Model file for the job. Use its own axes, mm. A direction names the side the tool comes from. Give positions to 0.01 mm unless a question says otherwise; leave off trailing zeros. Order: outer loops, then holes, each group sorted by start corner. A loop starts at its lowest first (then second) coordinate and runs counter-clockwise, first axis right, second up. Notation, with made-up numbers: (-31.75, 9.25) - (8.25, 9.25) arc R21 cw to (8.25, 45.25) - close; hole circle Ø9 at (32.25, 82.25). An arc over 180 degrees is marked (long way). Return JSON: item names as keys, results as strings. Group by question number.
from build123d import *

# Parameters (mm, degrees)
BOSS_EXTRUDE1_DEPTH      = 30
BOSS_EXTRUDE2_DEPTH      = 6.5
BOSS_EXTRUDE2_DEPTH_BACK = 6.5


with BuildPart() as part:
    # Sketch1 → Boss-Extrude1 (new body)
    with BuildSketch(Plane(origin=(0, 0, 0), x_dir=(1, 0, 0), z_dir=(0, 1, 0))):
        with BuildLine():
            Line((0, 66.57), (260, 66.57))
            ThreePointArc((260, 66.57), (326.57, 0), (260, -66.57))
            Line((260, -66.57), (0, -66.57))
            ThreePointArc((0, -66.57), (-66.57, 0), (0, 66.57))
        make_face()
        with BuildLine():
            Line((0, 58.57), (260, 58.57))
            ThreePointArc((260, 58.57), (318.57, 0), (260, -58.57))
            Line((260, -58.57), (0, -58.57))
            ThreePointArc((0, -58.57), (-58.57, 0), (0, 58.57))
        make_face(mode=Mode.SUBTRACT)
    extrude(amount=BOSS_EXTRUDE1_DEPTH)

    # Sketch2 → Boss-Extrude2 (add, two sides: drawn at the far end of the back side and taken through both)
    with BuildSketch(Plane(origin=(0, 15, 0), x_dir=(-1, 0, 0), z_dir=(0, -1, 0)).offset(-BOSS_EXTRUDE2_DEPTH_BACK)):
        with BuildLine():
            Line((0, -58.57), (-260, -58.57))
            ThreePointArc((-260, -58.57), (-318.57, 0), (-260, 58.57))
            Line((-260, 58.57), (0, 58.57))
            ThreePointArc((0, 58.57), (58.57, 0), (0, -58.57))
        make_face()
        with BuildLine():
            Line((0, -50.57), (-260, -50.57))
            ThreePointArc((-260, -50.57), (-310.57, 0), (-260, 50.57))
            Line((-260, 50.57), (0, 50.57))
            ThreePointArc((0, 50.57), (50.57, 0), (0, -50.57))
        make_face(mode=Mode.SUBTRACT)
    extrude(amount=BOSS_EXTRUDE2_DEPTH + BOSS_EXTRUDE2_DEPTH_BACK)


solid = part.part
(1) 3-axis set-ups, long thin cutter, end or side, ignore diameter. For faces 4 (the face through (326.554, 14.79, -1.464)), 5 (the face through (-58.556, 25.69, 1.288)), 6 (the face through (310.558, 15.091, 1.112)), 7 (the face through (-58.556, 4.19, 1.288)): which of +Z, -Z, +X, -X, +Y, -Y reach the whole face in a straight line?
(2) Drill centre lines: L1, parallel to Z at x = 125, y = 17; L2, parallel to Z at x = 26, y = 28; L3, parallel to Y at x = 81.5, z = 58.5. Where is each one in solid material? Low to high.
(3) Pull direction Z, two halves, no side cores. Call faces 1 (the face through (116, 30, 59)), 2 (the face through (-66.554, 14.79, 1.464)), 3 (the face through (318.556, 4.19, -1.288)): released by +Z, released by -Z, zero draft, split by the parting line, or undercut.
(4) Slice it at A-A (z = 0). Give the cut face in (x, y).
(5) Slice it at B-B (y = 13.5). Give the cut face in (x, z), and give its area (3 significant figures).
(6) Drop flat-ended pins along their axis: pin 1 Ø8 at (x, y) = (-10.5, 20) entering from +Z; pin 2 Ø12 at (y, z) = (26.5, -53) entering from +X; pin 3 Ø3 at (y, z) = (7, -13.5) entering from -X. Give the stop position or say it passes through.
(7) Slice it at C-C (x = 39.5). Give the cut face in (y, z).
Result set:
{
 "1": {"face 4": "+X, +Y, -Y", "face 5": "+Y", "face 6": "+Y, -Y", "face 7": "-Y"},
 "2": {"L1": "z = -66.57 to -50.57, 50.57 to 66.57", "L2": "z = -66.57 to -58.57, 58.57 to 66.57", "L3": "y = 8.5 to 21.5"},
 "3": {"face 1": "zero draft", "face 2": "split by the parting line", "face 3": "undercut"},
 "4": {"outline": "(-66.57, 0) - (-58.57, 0) - (-58.57, 8.5) - (-50.57, 8.5) - (-50.57, 21.5) - (-58.57, 21.5) - (-58.57, 30) - (-66.57, 30) - close; (310.57, 8.5) - (318.57, 8.5) - (318.57, 0) - (326.57, 0) - (326.57, 30) - (318.57, 30) - (318.57, 21.5) - (310.57, 21.5) - close"},
 "5": {"outline": "(0, -66.57) - (260, -66.57) arc R66.57 ccw to (260, 66.57) - (0, 66.57) arc R66.57 ccw to start; hole (0, -50.57) - (260, -50.57) arc R50.57 ccw to (260, 50.57) - (0, 50.57) arc R50.57 ccw to start", "area": "14,200 mm²"},
 "6": {"pin 1": "stops at z = 66.25", "pin 2": "stops at x = 307.14", "pin 3": "stops at x = -65.48"},
 "7": {"outline": "(0, -66.57) - (30, -66.57) - (30, -58.57) - (21.5, -58.57) - (21.5, -50.57) - (8.5, -50.57) - (8.5, -58.57) - (0, -58.57) - close; (0, 58.57) - (8.5, 58.57) - (8.5, 50.57) - (21.5, 50.57) - (21.5, 58.57) - (30, 58.57) - (30, 66.57) - (0, 66.57) - close"}
}
